Source: three-view drawing plus pictorial views. Frame: mm from the lowest corner of the part. A direction names the side the tool comes from. Coordinates: 2 decimals unless noted, no trailing zeros. Order: outer loops, then holes, each group sorted by start corner. A loop starts at its lowest first (then second) coordinate and runs counter-clockwise, first axis right, second up. Notation, with made-up numbers: M -27,86 L -22,86 A34 cw -22,121 Z; hole C -23,35.5 d2. An arc over 180 degrees is marked long. Use CSV: the item, a comma, the result in double quotes. Start each with the question number.
Q1. Section query C-C, the plane x = 10. Output: boundary loops of the cut face in (y, z), and give its area (3 significant figures).
Q2. Section query A-A, the plane x = 42.5. Output: boundary loops of the cut face in (y, z).
Q3. Ray query, probe 1 along Y at (x, z) = (97, 44); probe 2 along Z at (x, y) = (45.5, 20); probe 3 along X at (y, z) = (5, 32). Return the intervals inside material, ascending.
Q4. First-contact query: P1, Ø7.5, axis at y = 12.5, z = 34.5, coming from the -X side; P2, Ø7.5, axis at x = 49, y = 18, coming from the -Z side; P3, Ø10, axis at x = 17, y = 33.5, coming from the -Z side; P4, Ø7.5, axis at x = 40, y = 16, coming from the +Z side. Flat tips, straight axial feed; report the tip coordinate or a pass-through.
Q5. Access query for the marked faces 1, 2 and 3. Directions: +Z, -Z, +X, -X, +Y, -Y. A direction counts if a zero-diameter tool reaches every point of the face in a straight line with its end or side. Return the directions, or none.
Q6. Section query D-D, the plane z = 51.5. Output: boundary loops of the cut face in (x, y), and give its area (3 significant figures).
Q7. Section query B-B, the plane z = 29. Output: boundary loops of the cut face in (x, y), and give its area (3 significant figures).
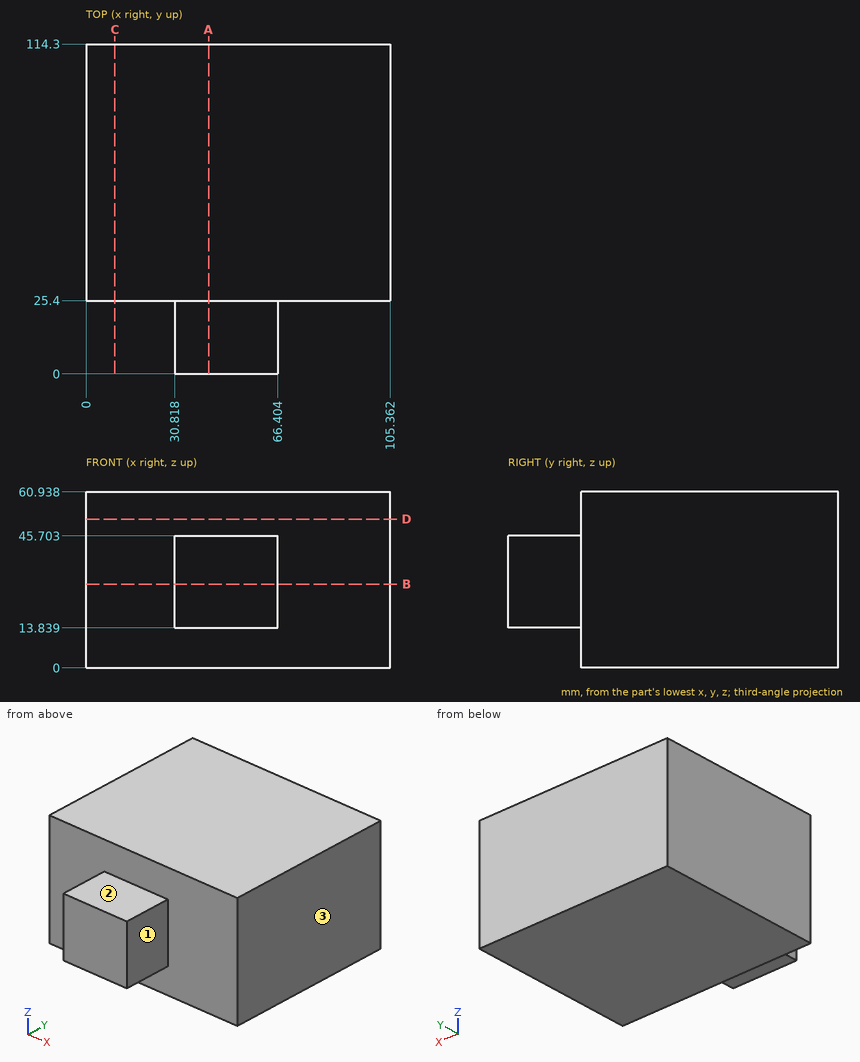
Responses:
1,outline,"M 25.4,0 L 114.3,0 L 114.3,60.94 L 25.4,60.94 Z"
1,area,"5,420 mm²"
2,outline,"M 0,13.84 L 25.4,13.84 L 25.4,0 L 114.3,0 L 114.3,60.94 L 25.4,60.94 L 25.4,45.7 L 0,45.7 Z"
3,probe 1,"y = 25.4 to 114.3"
3,probe 2,"z = 13.84 to 45.7"
3,probe 3,"x = 30.82 to 66.4"
4,P1,"stops at x = 30.82"
4,P2,"stops at z = 13.84"
4,P3,"stops at z = 0"
4,P4,"stops at z = 45.7"
5,face 1,"+Z, -Z, +X, -Y"
5,face 2,"+Z, +X, -X, -Y"
5,face 3,"+Z, -Z, +X, +Y, -Y"
6,outline,"M 0,25.4 L 105.36,25.4 L 105.36,114.3 L 0,114.3 Z"
6,area,"9,370 mm²"
7,outline,"M 0,25.4 L 30.82,25.4 L 30.82,0 L 66.4,0 L 66.4,25.4 L 105.36,25.4 L 105.36,114.3 L 0,114.3 Z"
7,area,"10,300 mm²"
